Part model, mm, in its own coordinate system. A direction names the side the tool comes from. Round coordinates to 2 decimals unless told otherwise and drop trailing zeros. Loops run counter-clockwise (first coordinate to the right, second up) from the corner with the lowest first, then second, coordinate; pieces in that order, holes last.
1) Band-saw the part on B-B, the plane z = 33. Write the cut outline in (x, y).
2) Band-saw the part on A-A, the plane y = 26. Write the cut outline in (x, z), then the cut area to 3 significant figures.
3) 3-axis set-ups, long thin cutter, end or side, ignore diameter. For faces 1 (the flat face through (0, 33, 4)), 2 (the flat face through (-7, 45.111, 26)), 3 (the flat face through (-14, 34.641, 3)), 4 (the flat face through (-14, 47, 36.788)), 5 (the flat face through (-29.997, 29, 18)): which of +Z, -Z, +X, -X, +Y, -Y reach the whole face in a straight line?
4) Band-saw the part on D-D, the plane y = 43.5. Write the cut outline in (x, z), then the cut area to 3 significant figures.
5) Drop flat-ended pins along their axis: P1, Ø1, axis at x = -22, y = 5.5, coming from the +Z side; P2, Ø10, axis at y = 38.5, z = 12, coming from the +X side; P3, Ø1.7, axis at y = 26, z = 3.5, coming from the +X side. Give the stop position or say it passes through.
6) Mould opens along Z. For faces 6 (the flat face through (-28.5, 21.4, 26.7)), 7 (the cylindrical face through (-18.341, 46.941, 36.064)), 8 (the cylindrical face through (-8.659, 15.285, 2.946)), 9 (the cylindrical face through (-9.95, 46.94, 19.5)) say: +Z half, -Z half, draft (parallel to the pull), parting line (faces both ways), or undercut.
7) Probe line 1 (Z direction, x = -14.25, y = 46); line 2 (X direction, y = 40.5, z = 16.5); line 3 (Y direction, x = -24, z = 6). List the from-to ranges inside material, lowest first.
8) Band-saw the part on C-C, the plane x = -15. Write the cut outline in (y, z), then the cut area to 3 significant figures.
from build123d import *

# Parameters (mm, degrees)
F1_DEPTH = 29.9974
F3_DEPTH = 27.0002
F6_DEPTH = 5.811617
F8_DEPTH = 3.712296


with BuildPart() as f1:
    # F0 (on Right) → F1 (new body)
    with BuildSketch(Plane.YZ):
        Polygon((0, 6.607804), (0, 0), (48.823252, 0), (48.823252, 46.265662), (42.241033, 46.265662), align=None)
    extrude(amount=-F1_DEPTH)


with BuildPart() as f3:
    # F2 (on Right) → F3 (new body)
    with BuildSketch(Plane.YZ):
        Polygon((45.110956, 5.811617), (45.110956, 61.896294), (-13.766318, 5.811617), align=None)
    extrude(amount=-F3_DEPTH)


with BuildPart() as f1_1:
    add(f1.part)

    # F4: cut F3
    add(f3.part, mode=Mode.SUBTRACT)

    # F5 (on face) → F6 (cut, through all)
    with BuildSketch(Plane.XY.offset(5.811617)):
        with BuildLine():
            Line((-10.435018, 34.640817), (-16.748959, 34.640817))
            ThreePointArc((-16.748959, 34.640817), (-18.54501, 33.896868), (-19.288959, 32.100817))
            Line((-19.288959, 32.100817), (-19.288959, 17.100303))
            ThreePointArc((-19.288959, 17.100303), (-18.54501, 15.304251), (-16.748959, 14.560303))
            Line((-16.748959, 14.560303), (-10.435018, 14.560303))
            ThreePointArc((-10.435018, 14.560303), (-8.638967, 15.304251), (-7.895018, 17.100303))
            Line((-7.895018, 17.100303), (-7.895018, 32.100817))
            ThreePointArc((-7.895018, 32.100817), (-8.638967, 33.896868), (-10.435018, 34.640817))
        make_face()
    extrude(amount=-F6_DEPTH, mode=Mode.SUBTRACT)

    # F7 (on face) → F8 (cut, through all)
    with BuildSketch(Plane.XZ.offset(-45.110956)):
        with BuildLine():
            Line((-11.721431, 36.788322), (-16.565181, 36.788322))
            ThreePointArc((-16.565181, 36.788322), (-18.361232, 36.044373), (-19.105181, 34.248322))
            Line((-19.105181, 34.248322), (-19.105181, 21.318551))
            ThreePointArc((-19.105181, 21.318551), (-18.361232, 19.5225), (-16.565181, 18.778551))
            Line((-16.565181, 18.778551), (-11.721431, 18.778551))
            ThreePointArc((-11.721431, 18.778551), (-9.925379, 19.5225), (-9.181431, 21.318551))
            Line((-9.181431, 21.318551), (-9.181431, 34.248322))
            ThreePointArc((-9.181431, 34.248322), (-9.925379, 36.044373), (-11.721431, 36.788322))
        make_face()
    extrude(amount=-F8_DEPTH, mode=Mode.SUBTRACT)


solid = f1_1.part
Reported:
1. outline: (-30, 28.11) - (-27, 28.11) - (-27, 45.11) - (-19.11, 45.11) - (-19.11, 48.82) - (-30, 48.82) - close; (-9.18, 45.11) - (0, 45.11) - (0, 48.82) - (-9.18, 48.82) - close
2. outline: (-30, 0) - (-19.29, 0) - (-19.29, 5.81) - (-27, 5.81) - (-27, 31.02) - (-30, 31.02) - close; (-7.9, 0) - (0, 0) - (0, 5.81) - (-7.9, 5.81) - close
2. area: 184 mm2
3. face 1: +Z, -Z, +X, +Y, -Y
3. face 2: +Z, +X, -Y
3. face 3: +Z, -Z
3. face 4: +Y, -Y
3. face 5: +Z, -Z, -X, +Y, -Y
4. outline: (-30, 0) - (0, 0) - (0, 5.81) - (-27, 5.81) - (-27, 46.27) - (-30, 46.27) - close
4. area: 296 mm2
5. P1: stops at z = 5.81
5. P2: stops at x = -27
5. P3: stops at x = 0
6. face 6: +Z half
6. face 7: undercut
6. face 8: draft
6. face 9: undercut
7. line 1: z = 0 to 18.78, 36.79 to 46.27
7. line 2: x = -30 to -27
7. line 3: y = 45.11 to 48.82
8. outline: (0, 0) - (14.56, 0) - (14.56, 5.81) - (0, 5.81) - close; (34.64, 0) - (48.82, 0) - (48.82, 18.78) - (45.11, 18.78) - (45.11, 5.81) - (34.64, 5.81) - close; (45.11, 36.79) - (48.82, 36.79) - (48.82, 46.27) - (45.11, 46.27) - close
8. area: 250 mm2
